For this review, take the finished solid that the model builds, in its own axes (mm). A direction names the side the tool comes from. Coordinates: 2 decimals unless noted, no trailing zeros. Loops run counter-clockwise (first coordinate to the right, second up) from the corner with the lowest first, then second, coordinate; pieces in that order, holes last. Notation, with made-up numbers: M 7,87 L 56,87 A22 ccw 56,94 Z; hole C 17,65 d1. An arc over 180 degrees is marked long. Write item = value, one per line.
from build123d import *

# Parameters (mm, degrees)
SKETCH1_W           = 30
SKETCH1_H           = 9
BOSS_EXTRUDE1_DEPTH = 9
SKETCH3_R           = 2.75
CUT_EXTRUDE1_DEPTH  = 113.202955527


with BuildPart() as part:
    # Sketch1 → Boss-Extrude1 (new body)
    with BuildSketch(Plane(origin=(0, 0, 0), x_dir=(1, 0, 0), z_dir=(0, 1, 0))):
        Polygon((50, -88.042507111), (50, -68.042507111), (41, -68.042507111), (41, -56.042507111), (35, -56.042507111), (35, -47.042507111), (50, -47.042507111), (50, -33), (-50, -33), (-50, -47.042507111), (-35, -47.042507111), (-35, -56.042507111), (-41, -56.042507111), (-41, -68.042507111), (-50, -68.042507111), (-50, -88.042507111), (-41, -88.042507111), (-41, -100.042507111), (41, -100.042507111), (41, -88.042507111), align=None)
        with Locations((0, -51.542507111)):
            Rectangle(SKETCH1_W, SKETCH1_H, mode=Mode.SUBTRACT)
    extrude(amount=BOSS_EXTRUDE1_DEPTH)

    # Sketch3 → Cut-Extrude1 (cut, through all)
    with BuildSketch(Plane(origin=(0, 9, 0), x_dir=(1, 0, 0), z_dir=(0, 1, 0))):
        with Locations(Location((-45, -40, 0), (0, 0, 270))):
            Circle(SKETCH3_R)
        with Locations(Location((-13, -40, 0), (0, 0, 270))):
            Circle(SKETCH3_R)
        with Locations(Location((13, -40, 0), (0, 0, 90))):
            Circle(SKETCH3_R)
        with Locations(Location((45, -40, 0), (0, 0, 90))):
            Circle(SKETCH3_R)
    extrude(amount=-CUT_EXTRUDE1_DEPTH, mode=Mode.SUBTRACT)


solid = part.part
Q1. Add section A-A (z = 53). Write out the cut boundary in (x, y).
Solved:
outline = M -35,0 L -15,0 L -15,9 L -35,9 Z; M 15,0 L 35,0 L 35,9 L 15,9 Z
Q2. For line 1 along X through (y, z) = (7, 40); line 2 along Z through (x, y) = (13, 6.5); line 3 along X through (y, z) = (6.5, 50.5), list the stretches that pass through material, from the lowest coordinate up.
Solved:
line_1 = -50 to -47.75, -42.25 to -15.75, -10.25 to 10.25, 15.75 to 42.25, 47.75 to 50
line_2 = 33 to 37.25, 42.75 to 47.04, 56.04 to 100.04
line_3 = -35 to -15, 15 to 35
Q3. Add section C-C (x = -45). Write out the cut boundary in (y, z).
Solved:
outline = M 0,33 L 9,33 L 9,37.25 L 0,37.25 Z; M 0,42.75 L 9,42.75 L 9,47.04 L 0,47.04 Z; M 0,68.04 L 9,68.04 L 9,88.04 L 0,88.04 Z
Q4. Add section B-B (x = -4.5). Write out the cut boundary in (y, z), and give its area (3 significant figures).
Solved:
outline = M 0,33 L 9,33 L 9,47.04 L 0,47.04 Z; M 0,56.04 L 9,56.04 L 9,100.04 L 0,100.04 Z
area = 522 mm²
Q5. For pin 1 Ø1.5 at (y, z) = (7.5, 61) entering from +X; pin 2 Ø1.5 at (y, z) = (2.5, 58.5) entering from -X; pin 3 Ø4.5 at (y, z) = (3, 51) entering from -X, all flat-tipped, find the tip position at first contact; note any pin that passes through.
Solved:
pin_1 = 41
pin_2 = -41
pin_3 = -35
Q6. Add section D-D (y = 2.75). Write out the cut boundary in (x, z).
Solved:
outline = M -50,33 L 50,33 L 50,47.04 L 35,47.04 L 35,56.04 L 41,56.04 L 41,68.04 L 50,68.04 L 50,88.04 L 41,88.04 L 41,100.04 L -41,100.04 L -41,88.04 L -50,88.04 L -50,68.04 L -41,68.04 L -41,56.04 L -35,56.04 L -35,47.04 L -50,47.04 Z; hole C -45,40 d5.5; hole C -13,40 d5.5; hole M -15,47.04 L 15,47.04 L 15,56.04 L -15,56.04 Z; hole C 13,40 d5.5; hole C 45,40 d5.5
Q7. Draft analysis for pull direction X (two halves, no side actions). For faces 4 (the face through (0, 4, 56.043)), 5 (the face through (41, 4, 62)), 6 (the face through (38, 4, 56.043)), state which applies: +X half, -X half, draft (parallel to the pull), parting line (faces both ways), or undercut.
Solved:
face_4 = undercut
face_5 = +X half
face_6 = draft
Q8. Machinability: for faces 1 (the face through (-41, 4, 62)), 2 (the face through (-41, 4, 94)), 3 (the face through (35, 4, 52)), which of the approach directions +Z, -Z, +X, -X, +Y, -Y give a long, thin tool a straight path to every point of the face, cutting with its end or side? Answer none if there is none.
Solved:
face_1 = -X, +Y, -Y
face_2 = +Z, -X, +Y, -Y
face_3 = +X, +Y, -Y
